```python
from build123d import *

# Parameters (mm, degrees)
BOSS_EXTRUDE1_DEPTH = 2.3
CUT_EXTRUDE1_START  = 25
SKETCH2_R           = 0.675
CUT_EXTRUDE1_DEPTH  = 12.5
BOSS_EXTRUDE2_START = 34
SKETCH2_8_R         = 0.675
BOSS_EXTRUDE2_DEPTH = 1.5
BOSS_EXTRUDE5_START = 14.5
SKETCH2_11_R        = 0.675
BOSS_EXTRUDE5_DEPTH = 1.5
BOSS_EXTRUDE3_START = 10.5
SKETCH4_R           = 0.825
BOSS_EXTRUDE3_DEPTH = 1


with BuildPart() as part:
    # Sketch1 → Boss-Extrude1 (new body)
    with BuildSketch(Plane(origin=(0, 0, 0), x_dir=(1, 0, 0), z_dir=(0, 1, 0))):
        with BuildLine():
            ThreePointArc((48.989794856, 25), (0, 55), (-48.989794856, 25))
            Line((-48.989794856, 25), (48.989794856, 25))
        make_face()
    extrude(amount=BOSS_EXTRUDE1_DEPTH)

    # Sketch2 → Cut-Extrude1 (cut, symmetric)
    with BuildSketch(Plane(origin=(0, 0, 0), x_dir=(0, 0, -1), z_dir=(1, 0, 0)).offset(CUT_EXTRUDE1_START)):
        with BuildLine():
            Line((25, 0), (26.991919376, 0))
            ThreePointArc((26.991919376, 0), (27.634812595, 1.15), (26.991919376, 2.3))
            Line((26.991919376, 2.3), (25, 2.3))
            Line((25, 2.3), (25, 0))
        make_face()
        with Locations((26.284812595, 1.15)):
            Circle(SKETCH2_R, mode=Mode.SUBTRACT)
        with Locations((26.284812595, 1.15)):
            Circle(SKETCH2_R)
    cut_extrude1 = extrude(amount=CUT_EXTRUDE1_DEPTH, both=True, mode=Mode.SUBTRACT)

    # Sketch2_8 → Boss-Extrude2 (add)
    with BuildSketch(Plane(origin=(0, 0, 0), x_dir=(0, 0, -1), z_dir=(1, 0, 0)).offset(BOSS_EXTRUDE2_START)):
        with BuildLine():
            Line((25, 0), (26.991919376, 0))
            ThreePointArc((26.991919376, 0), (27.634812595, 1.15), (26.991919376, 2.3))
            Line((26.991919376, 2.3), (25, 2.3))
            Line((25, 2.3), (25, 0))
        make_face()
        with Locations((26.284812595, 1.15)):
            Circle(SKETCH2_8_R, mode=Mode.SUBTRACT)
    boss_extrude2 = extrude(amount=BOSS_EXTRUDE2_DEPTH)

    # Sketch2_11 → Boss-Extrude5 (add)
    with BuildSketch(Plane(origin=(0, 0, 0), x_dir=(0, 0, -1), z_dir=(1, 0, 0)).offset(BOSS_EXTRUDE5_START)):
        with BuildLine():
            Line((25, 0), (26.991919376, 0))
            ThreePointArc((26.991919376, 0), (27.634812595, 1.15), (26.991919376, 2.3))
            Line((26.991919376, 2.3), (25, 2.3))
            Line((25, 2.3), (25, 0))
        make_face()
        with Locations((26.284812595, 1.15)):
            Circle(SKETCH2_11_R, mode=Mode.SUBTRACT)
    boss_extrude5 = extrude(amount=BOSS_EXTRUDE5_DEPTH)

    # Mirror1: Cut-Extrude1, Boss-Extrude2, Boss-Extrude5 across plane
    add(cut_extrude1.mirror(Plane(origin=(0, 0, 0), x_dir=(0, 0, 1), z_dir=(1, 0, 0))), mode=Mode.SUBTRACT)
    add(boss_extrude2.mirror(Plane(origin=(0, 0, 0), x_dir=(0, 0, 1), z_dir=(1, 0, 0))))
    add(boss_extrude5.mirror(Plane(origin=(0, 0, 0), x_dir=(0, 0, 1), z_dir=(1, 0, 0))))

    # Sketch4 → Boss-Extrude3 (add, symmetric)
    with BuildSketch(Plane(origin=(0, 0, 0), x_dir=(0, 0, -1), z_dir=(1, 0, 0)).offset(BOSS_EXTRUDE3_START)):
        with BuildLine():
            Line((41.125, 0), (38.875, 0))
            Line((38.875, 0), (38.875, -1.8))
            ThreePointArc((38.875, -1.8), (40, -2.925), (41.125, -1.8))
            Line((41.125, -1.8), (41.125, 0))
        make_face()
        with Locations((40, -1.8)):
            Circle(SKETCH4_R, mode=Mode.SUBTRACT)
    extrude(amount=BOSS_EXTRUDE3_DEPTH, both=True)


solid = part.part
```
Verification items for the finished model (mm, model axes). A direction names the side the tool comes from. Coordinates: 2 decimals unless noted, no trailing zeros. Loops run counter-clockwise (first coordinate to the right, second up) from the corner with the lowest first, then second, coordinate; pieces in that order, holes last. Notation, with made-up numbers: (-14, 37.25) - (38, 37.25) arc R22 ccw to (38, 63.25) - close; hole circle Ø2 at (12.25, 63). An arc over 180 degrees is marked (long way). Answer as a JSON object with one key per item and string values.
(1) Mould release check, pull along Y, two halves, no side actions. Record for faces 1 (the flat face through (-1, 2.3, -37)), 2 (the flat face through (9.5, -0.8, -40)), 3 (the flat face through (-16, 2, -26)): pulls with the +Y half, pulls with the -Y half, needs draft (parallel to the pull), parting line crosses it, or undercut.
Response:
{"face 1": "pulls with the +Y half", "face 2": "needs draft", "face 3": "undercut"}
(2) Go/stop test with flat-tipped pins: pin 1 Ø1.4 at (x, y) = (10.5, -1) entering from +Z (3 decimals); pin 2 Ø2 at (x, z) = (-3.5, -39) entering from -Y; pin 3 Ø1.1 at (y, z) = (1.15, -26.28) entering from -X. Record where each tip stops, or that it passes through.
Response:
{"pin 1": "stops at z = -38.875", "pin 2": "stops at y = 0", "pin 3": "stops at x = -48.61"}
(3) Cross-section at C-C, the plane z = -47. Record the boundary of the cut face in (x, y).
Response:
{"outline": "(-28.57, 0) - (28.57, 0) - (28.57, 2.3) - (-28.57, 2.3) - close"}
(4) Cross-section at A-A, the plane z = -40. Record the boundary of the cut face in (x, y) (3 decimals).
Response:
{"outline": "(-37.749, 0) - (9.5, 0) - (9.5, -0.975) - (11.5, -0.975) - (11.5, 0) - (37.749, 0) - (37.749, 2.3) - (-37.749, 2.3) - close; (9.5, -2.925) - (11.5, -2.925) - (11.5, -2.625) - (9.5, -2.625) - close"}
(5) Scan lines: line 1 along Y through (x, z) = (10, -40) (3 decimals); line 2 along Y through (x, z) = (35.5, -33.5); line 3 along X through (y, z) = (0.55, -35.5). Record each from-to range of solid material in increasing order.
Response:
{"line 1": "y = -2.925 to -2.625, -0.975 to 2.3", "line 2": "y = 0 to 2.3", "line 3": "x = -42.01 to 42.01"}
(6) Access from +Z, -Z, +X, -X, +Y, -Y to the whole of each face (thin tool, end or side, straight path). Record for faces 4 (the cylindrical face through (0.846, 1.134, -54.993)), 5 (the flat face through (34, 2, -26)).
Response:
{"face 4": "-Z, +Y, -Y", "face 5": "+Z"}
(7) Cross-section at B-B, the plane x = -31. Record the boundary of the cut face in (y, z), then the cut area to 3 significant figures.
Response:
{"outline": "(0, -45.43) - (2.3, -45.43) - (2.3, -26.99) arc R1.35 cw to (0, -26.99) - close", "area": "41.4 mm²"}
